```python
from build123d import *

# Parameters (mm, degrees)
TAPPED_HOLE1_D     = 2.5
TAPPED_HOLE1_DEPTH = 8.5
TAPPED_HOLE1_TIP   = 0.751075774
TAPPED_HOLE2_D     = 2.5
TAPPED_HOLE2_DEPTH = 8.5
TAPPED_HOLE2_TIP   = 0.751075774
CHAMFER1_SIZE      = 0.2
CHAMFER2_SIZE      = 0.2
CHAMFER3_SIZE      = 0.5


with BuildPart() as part:
    # Sketch1 → Revolve1 (revolve)
    with BuildSketch(Plane.XY, mode=Mode.PRIVATE) as revolve1_sk:
        Polygon((0, 0), (114, 0), (114, 2.5), (111.5, 2.5), (111.5, 3), (2.5, 3), (2.5, 2.5), (0, 2.5), align=None)
    revolve(revolve1_sk.sketch.rotate(Axis((0, 0, 0), (1, 0, 0)), 90), axis=Axis((0, 0, 0), (1, 0, 0)))

    # Tapped Hole1
    with Locations(Plane.ZY):
        with Locations((0, 0)):
            Hole(TAPPED_HOLE1_D / 2, depth=TAPPED_HOLE1_DEPTH)
            with Locations((0, 0, -(TAPPED_HOLE1_DEPTH + TAPPED_HOLE1_TIP / 2))):  # 118° drill point
                Cone(0, TAPPED_HOLE1_D / 2, TAPPED_HOLE1_TIP, mode=Mode.SUBTRACT)

    # Tapped Hole2
    with Locations(Plane(origin=(114, 0, 0), x_dir=(0, 0, -1), z_dir=(1, 0, 0))):
        with Locations((0, 0)):
            Hole(TAPPED_HOLE2_D / 2, depth=TAPPED_HOLE2_DEPTH)
            with Locations((0, 0, -(TAPPED_HOLE2_DEPTH + TAPPED_HOLE2_TIP / 2))):  # 118° drill point
                Cone(0, TAPPED_HOLE2_D / 2, TAPPED_HOLE2_TIP, mode=Mode.SUBTRACT)

    # Chamfer1
    chamfer1_edges = [part.edges().sort_by_distance(p)[0] for p in [
        (111.5, 0, -3),
    ]]
    chamfer(chamfer1_edges, length=CHAMFER1_SIZE)

    # Chamfer2
    chamfer2_edges = [part.edges().sort_by_distance(p)[0] for p in [
        (2.5, 0, -3),
    ]]
    chamfer(chamfer2_edges, length=CHAMFER2_SIZE)

    # Chamfer3
    chamfer3_edges = [part.edges().sort_by_distance(p)[0] for p in [
        (0, 0, -2.5),
        (114, 0, -2.5),
    ]]
    chamfer(chamfer3_edges, length=CHAMFER3_SIZE)


solid = part.part
```
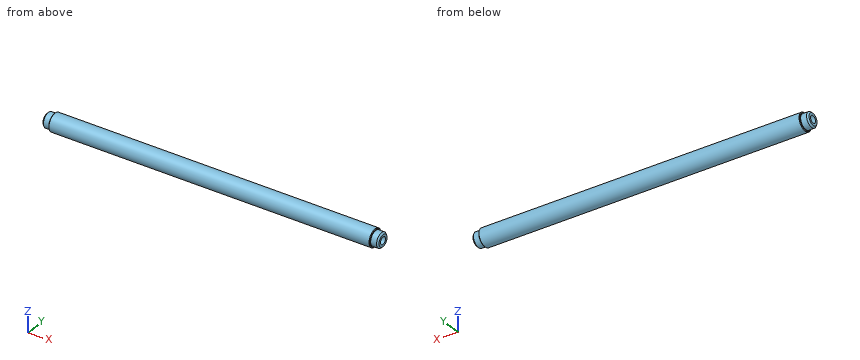
Source: CAD feature listing. Evaluate the final solid. Frame: model axes, mm. Round coordinates to 2 decimals unless told otherwise and drop trailing zeros. Loops run counter-clockwise (first coordinate to the right, second up) from the corner with the lowest first, then second, coordinate; pieces in that order, holes last.
(1) Section query A-A (x = 93.5). Output: boundary loops of the cut face in (y, z).
From the geometry:
outline: circle Ø6 at (0, 0)
(2) Material intervals for probe 1 along Y at (x, z) = (109.5, 0); probe 2 along Y at (x, z) = (2, 0); probe 3 along Y at (x, z) = (47, -1.1), sorted ascending.
From the geometry:
probe 1: y = -3 to -1.25, 1.25 to 3
probe 2: y = -2.5 to -1.25, 1.25 to 2.5
probe 3: y = -2.79 to 2.79
(3) Contact query for flat-ended pins moving along their axis: pin 1 Ø2 at (y, z) = (-1, -1.5) entering from -X; pin 2 Ø2 at (x, y) = (18.5, 1.5) entering from +Z; pin 3 Ø3 at (x, z) = (60, 2) entering from -Y; pin 4 Ø2 at (y, z) = (0, 0) entering from -X. Output: stop coordinate, or through.
From the geometry:
pin 1: stops at x = 0
pin 2: stops at z = 2.96
pin 3: stops at y = -2.96
pin 4: stops at x = 8.65
